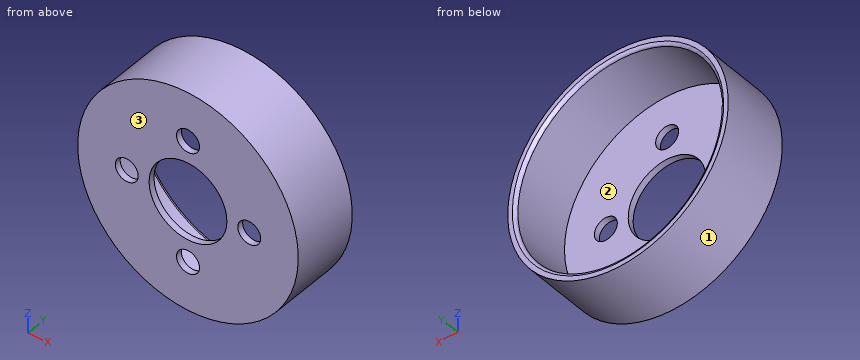
from build123d import *

# Parameters (mm, degrees)
SKETCH1_R           = 45.72
SKETCH1_R_2         = 42.545
BOSS_EXTRUDE1_DEPTH = 2.54
SKETCH2_R           = 45.72
SKETCH2_R_2         = 42.545
BOSS_EXTRUDE2_DEPTH = 25.4
CUT_EXTRUDE1_REACH  = 72.436
SKETCH3_R           = 16.129
FILLET1_R           = 1.27
CUT_EXTRUDE2_REACH  = 71.468
SKETCH5_R           = 4.7625
CIRPATTERN1_COUNT   = 4


with BuildPart() as part:
    # Sketch1 → Boss-Extrude1 (new body)
    # profile 1 of 2: a face of its own
    with BuildSketch(Plane(origin=(0, 0, 0), x_dir=(1, 0, 0), z_dir=(0, 1, 0))):
        with Locations(Location((0, 0, 0), (0, 0, 270))):
            Circle(SKETCH1_R)
        Circle(SKETCH1_R_2, mode=Mode.SUBTRACT)
    # profile 2 of 2: a face of its own
    with BuildSketch(Plane(origin=(0, 0, 0), x_dir=(1, 0, 0), z_dir=(0, 1, 0))):
        Circle(SKETCH1_R_2)
    extrude(amount=BOSS_EXTRUDE1_DEPTH)

    # Sketch2 → Boss-Extrude2 (add)
    with BuildSketch(Plane(origin=(0, 2.54, 0), x_dir=(1, 0, 0), z_dir=(0, 1, 0))):
        with Locations(Location((0, 0, 0), (0, 0, 270))):
            Circle(SKETCH2_R)
        with Locations(Location((0, 0, 0), (0, 0, 270))):
            Circle(SKETCH2_R_2, mode=Mode.SUBTRACT)
    extrude(amount=BOSS_EXTRUDE2_DEPTH)

    # Sketch3 → Cut-Extrude1 (cut, up to next)
    with BuildSketch(Plane.XZ, mode=Mode.PRIVATE) as cut_extrude1_sk1:
        with Locations(Location((0, 0, 0), (0, 0, 270))):
            Circle(SKETCH3_R)
    cut_extrude1_tool1 = extrude(cut_extrude1_sk1.sketch, amount=-CUT_EXTRUDE1_REACH, mode=Mode.PRIVATE) & part.part
    add(cut_extrude1_tool1.solids().sort_by_distance((0, 0, 0))[0], mode=Mode.SUBTRACT)

    # Fillet1
    fillet1_edges = [part.edges().sort_by_distance(p)[0] for p in [
        (0, 27.94, -42.545),
    ]]
    fillet(fillet1_edges, radius=FILLET1_R)

    # Sketch5 → Cut-Extrude2 (cut, up to next)
    with BuildSketch(Plane(origin=(0, 2.54, 0), x_dir=(1, 0, 0), z_dir=(0, 1, 0)), mode=Mode.PRIVATE) as cut_extrude2_sk1:
        with Locations(Location((0, 25.4, 0), (0, 0, 270))):
            Circle(SKETCH5_R)
    cut_extrude2_tool1 = extrude(cut_extrude2_sk1.sketch, amount=-CUT_EXTRUDE2_REACH, mode=Mode.PRIVATE) & part.part
    cut_extrude2 = cut_extrude2_tool1.solids().sort_by_distance((0, 2.54, -25.4))[0]
    add(cut_extrude2, mode=Mode.SUBTRACT)

    # CirPattern1: Cut-Extrude2 ×4 about axis
    cirpattern1_axis = Axis((0, 0, 0), (0, 1, 0))
    for i in range(1, CIRPATTERN1_COUNT):
        add(cut_extrude2.rotate(cirpattern1_axis, i * 360 / CIRPATTERN1_COUNT), mode=Mode.SUBTRACT)


solid = part.part
Geometry check sheet. Reference: the model listing, model coordinates, mm. Face numbers are marked on the shaded views. Give positions to 0.01 mm unless a question says otherwise; leave off trailing zeros. Loops run counter-clockwise (first coordinate to the right, second up) from the corner with the lowest first, then second, coordinate; pieces in that order, holes last. Notation, with made-up numbers: (42.5, 86.25) -> (46.5, 86.25) arc R22 ccw to (46.5, 92.25) -> close; hole circle Ø6 at (88, -13.75). An arc over 180 degrees is marked (long way). Answer in a Markdown table with one row per item. Add a question column.
1) Material ranges on probe 1 along Z at (x, y) = (-0.5, 5.25); probe 2 along Y at (x, z) = (-34, -22.5); probe 3 along Z at (x, y) = (-4.5, 23.75), recorded low to high. Write a range as from..to.
2) Cross-section at B-B on x = 0. Record the boundary of the cut face in (y, z) (1 decimal).
3) Cross-section at A-A on z = 0. Record the boundary of the cut face in (x, y) (1 decimal), and give its area (3 significant figures).
4) Draft check along Z on the marked faces 1, 2 and 3. Enter one of: pulls with the +Z half, pulls with the -Z half, needs draft (parallel to the pull), parting line crosses it, or undercut.
5) Cross-section at C-C on y = 20.5. Record the boundary of the cut face in (x, z) (3 decimals), and give its area (3 significant figures).
6) Gauge pin test, flat ends, axial feed: P1, Ø12, axis at x = 12.5, z = -23, coming from the +Y side; P2, Ø2, axis at x = -6.5, y = 17.5, coming from the +Z side; P3, Ø1, axis at y = 4, z = -21, coming from the -X side; P4, Ø5.5, axis at x = 25.4, z = 0, coming from the -Y side. Record the tip position at first contact, or that the pin passes through.
Outcome:
| question | item | result |
|---|---|---|
| 1 | probe 1 | z = -45.72..-42.54, 42.54..45.72 |
| 1 | probe 2 | y = 0..2.54 |
| 1 | probe 3 | z = -45.5..-42.31, 42.31..45.5 |
| 2 | outline | (0, -45.7) -> (27.9, -45.7) -> (27.9, -43.8) arc R1.3 ccw to (26.7, -42.5) -> (2.5, -42.5) -> (2.5, -30.2) -> (0, -30.2) -> close; (0, -20.6) -> (2.5, -20.6) -> (2.5, -16.1) -> (0, -16.1) -> close; (0, 16.1) -> (2.5, 16.1) -> (2.5, 20.6) -> (0, 20.6) -> close; (0, 30.2) -> (2.5, 30.2) -> (2.5, 42.5) -> (26.7, 42.5) arc R1.3 ccw to (27.9, 43.8) -> (27.9, 45.7) -> (0, 45.7) -> close |
| 3 | outline | (-45.7, 0) -> (-30.2, 0) -> (-30.2, 2.5) -> (-42.5, 2.5) -> (-42.5, 26.7) arc R1.3 ccw to (-43.8, 27.9) -> (-45.7, 27.9) -> close; (-20.6, 0) -> (-16.1, 0) -> (-16.1, 2.5) -> (-20.6, 2.5) -> close; (16.1, 0) -> (20.6, 0) -> (20.6, 2.5) -> (16.1, 2.5) -> close; (30.2, 0) -> (45.7, 0) -> (45.7, 27.9) -> (43.8, 27.9) arc R1.3 ccw to (42.5, 26.7) -> (42.5, 2.5) -> (30.2, 2.5) -> close |
| 3 | area | 263 mm^2 |
| 4 | face 1 | parting line crosses it |
| 4 | face 2 | undercut |
| 4 | face 3 | needs draft |
| 5 | outline | circle Ø91.44 at (0, 0); hole circle Ø85.09 at (0, 0) |
| 5 | area | 880 mm^2 |
| 6 | P1 | stops at y = 2.54 |
| 6 | P2 | stops at z = 45.39 |
| 6 | P3 | stops at x = -40.87 |
| 6 | P4 | passes through |
